```python
from build123d import *

# Parameters (mm, degrees)
HEXDIESKE_R  = 3.7125
HEXDIE_DEPTH = 0.4312


with BuildPart() as part:
    # BodySke → Body (revolve)
    with BuildSketch(Plane.XY, mode=Mode.PRIVATE) as body_sk:
        Polygon((2.695, 0), (3.712, 0), (3.712, 0.4312), (2.695, 0.4312), (2.4255, 0.586795898), (2.4255, 0.88396), (2.695, 0.88396), (2.695, 14), (1.45, 14), (1.45, 7), (0, 7), (0, 0.00254), (2.695, 0.00254), align=None)
    revolve(body_sk.sketch.rotate(Axis((0, 0, 0), (0, 1, 0)), 90), axis=Axis((0, 0, 0), (0, 1, 0)))

    # TapDriSke → TapDrill (revolve, cut)
    with BuildSketch(Plane.XY, mode=Mode.PRIVATE) as tapdrill_sk:
        Polygon((1.45, 4), (1.45, 14), (0, 14), (0, 3.399390335), align=None)
    revolve(tapdrill_sk.sketch.rotate(Axis((0, 0, 0), (0, 1, 0)), 90), axis=Axis((0, 0, 0), (0, 1, 0)), mode=Mode.SUBTRACT)

    # EndChamferSke → EndChamfer (revolve, cut)
    with BuildSketch(Plane.XY, mode=Mode.PRIVATE) as endchamfer_sk:
        Polygon((1.7515, 13.99746), (1.7515, 14.254), (1.45, 14.254), (1.45, 13.78747576), (1.75, 13.99746), align=None)
    revolve(endchamfer_sk.sketch.rotate(Axis((0, -2.54, 0), (0, 1, 0)), 90), axis=Axis((0, -2.54, 0), (0, 1, 0)), mode=Mode.SUBTRACT)

    # HexDieSke → HexDie (cut)
    with BuildSketch(Plane(origin=(0, 0.4312, 0), x_dir=(-1, 0, 0), z_dir=(0, 1, 0))):
        Circle(HEXDIESKE_R)
        Polygon((0, 3.695041723), (3.2, 1.847520861), (3.2, -1.847520861), (0, -3.695041723), (-3.2, -1.847520861), (-3.2, 1.847520861), align=None, mode=Mode.SUBTRACT)
    extrude(amount=-HEXDIE_DEPTH, mode=Mode.SUBTRACT)


solid = part.part
```
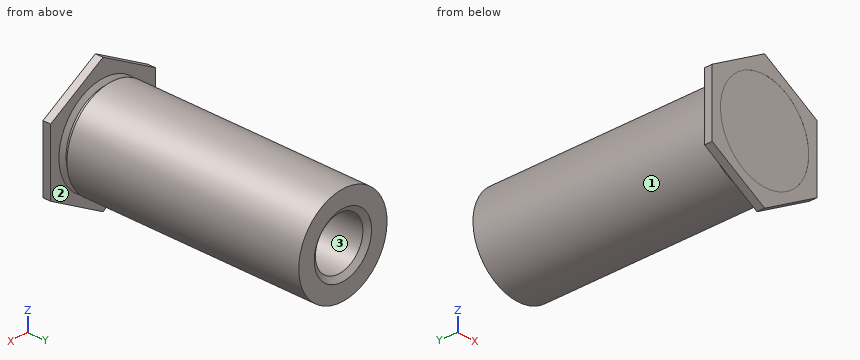
Model file for the job. Use its own axes, mm. Face numbers are marked on the shaded views. Coordinates: 2 decimals unless noted, no trailing zeros. Order: outer loops, then holes, each group sorted by start corner. A loop starts at its lowest first (then second) coordinate and runs counter-clockwise, first axis right, second up. Notation, with made-up numbers: (41.25, 85.25) -> (78.25, 85.25) arc R9 ccw to (78.25, 97.25) -> close; hole circle Ø11 at (-14.5, 24). An arc over 180 degrees is marked (long way). Answer as a JSON object with one key per item and string values. Group by question number.
1) Cut at B-B, the plane z = 3. Write the cut outline in (x, y), then the cut area to 3 significant figures.
2) Drill centre lines: L1, parallel to X at y = 7.5, z = 0 (3 decimals); L2, parallel to Y at x = -2.75, z = 0; L3, parallel to Y at x = -1.5, z = -2. Where is each one in solid material? Low to high.
3) Pull direction X, two halves, no side cores. Call the marked faces 1, 2 and 3: +X half, -X half, draft (parallel to the pull), parting line (faces both ways), or undercut.
4) Cut at A-A, the plane y = 7.5. Write the cut outline in (x, z) (3 decimals).
5) Flat gauge pins, fed straight in: pin 1 (1.5 mm diameter, centred on x = -1, z = 1, fed in from -Y); pin 2 (1 mm diameter, centred on x = 1.5, y = 5.5, fed in from +Z); pin 3 (1 mm diameter, centred on x = 1, z = 0, fed in from +Y); pin 4 (3 mm diameter, centred on x = 1, z = -1, fed in from +Y). Where does each tip first touch, or does it go through?
Check values:
{
 "1": {"outline": "(-1.2, 0) -> (1.2, 0) -> (1.2, 0.43) -> (-1.2, 0.43) -> close", "area": "1.04 mm²"},
 "2": {"L1": "x = -2.695 to -1.45, 1.45 to 2.695", "L2": "y = 0 to 0.43", "L3": "y = 0 to 0.54, 0.88 to 14"},
 "3": {"face 1": "parting line", "face 2": "draft", "face 3": "undercut"},
 "4": {"outline": "circle Ø5.39 at (0, 0); hole circle Ø2.9 at (0, 0)"},
 "5": {"pin 1": "stops at y = 0", "pin 2": "stops at z = 2.5", "pin 3": "stops at y = 13.82", "pin 4": "stops at y = 14"}
}
